from build123d import *

# Parameters (mm, degrees)
BOSS_EXTRUDE1_DEPTH      = 38.735
BOSS_EXTRUDE1_DEPTH_BACK = 38.735
CUT_EXTRUDE4_DEPTH       = 40.625695711


with BuildPart() as part:
    # Sketch1 → Boss-Extrude1 (new, two sides: drawn at the far end of the back side and taken through both)
    with BuildSketch(Plane(origin=(0, 0, 0), x_dir=(1, 0, 0), z_dir=(0, 1, 0)).offset(-BOSS_EXTRUDE1_DEPTH_BACK)):
        with BuildLine():
            Line((2.3876, 4.120773288), (-2.3876, 4.120773288))
            ThreePointArc((-2.3876, 4.120773288), (-2.378072881, -4.126278665), (4.7625, 0))
            ThreePointArc((4.7625, 0), (4.126278665, 2.378072881), (2.3876, 4.120773288))
        make_face()
    extrude(amount=BOSS_EXTRUDE1_DEPTH + BOSS_EXTRUDE1_DEPTH_BACK)

    # Sketch4 → Cut-Extrude4 (cut, through all)
    with BuildSketch(Plane.XY.offset(2.7432)):
        with BuildLine():
            Line((-1.2446, -26.035), (-1.2446, -38.735))
            Line((-1.2446, -38.735), (1.2446, -38.735))
            Line((1.2446, -38.735), (1.2446, -26.035))
            ThreePointArc((1.2446, -26.035), (0, -27.2796), (-1.2446, -26.035))
        make_face()
        with BuildLine():
            ThreePointArc((1.2446, -26.035), (0, -24.7904), (-1.2446, -26.035))
            Line((-1.2446, -26.035), (1.2446, -26.035))
        make_face()
        with BuildLine():
            Line((1.2446, -26.035), (-1.2446, -26.035))
            ThreePointArc((-1.2446, -26.035), (0, -27.2796), (1.2446, -26.035))
        make_face()
        with BuildLine():
            Line((1.2446, 38.735), (-1.2446, 38.735))
            Line((-1.2446, 38.735), (-1.2446, 26.035))
            ThreePointArc((-1.2446, 26.035), (0, 27.2796), (1.2446, 26.035))
            Line((1.2446, 26.035), (1.2446, 38.735))
        make_face()
        with BuildLine():
            ThreePointArc((1.2446, 26.035), (0, 27.2796), (-1.2446, 26.035))
            Line((-1.2446, 26.035), (1.2446, 26.035))
        make_face()
        with BuildLine():
            Line((1.2446, 26.035), (-1.2446, 26.035))
            ThreePointArc((-1.2446, 26.035), (0, 24.7904), (1.2446, 26.035))
        make_face()
    extrude(amount=CUT_EXTRUDE4_DEPTH, mode=Mode.SUBTRACT)


solid = part.part
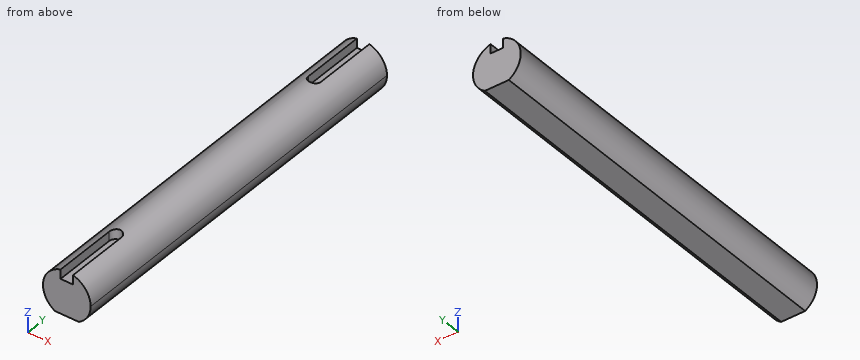
Here's how the part is built. I have some questions about the finished solid (model axes, mm). Round coordinates to 2 decimals unless told otherwise and drop trailing zeros. Loops run counter-clockwise (first coordinate to the right, second up) from the corner with the lowest first, then second, coordinate; pieces in that order, holes last. Notation, with made-up numbers: M -37.75,68.25 L 9.25,68.25 A24 cw 9.25,102.25 Z; hole C -26.75,56 d2. An arc over 180 degrees is marked long. Write each question's results on one line, items separated by ' | '. Start each with the question number.
(1) I want a section at D-D (y = -22.5). Please give me the cut outline in (x, z) (1 decimal).
(2) Will these pins go through, and if not, where does the flat tip stop? P1, Ø2, axis at y = 29.5, z = 1.5, coming from the +X side; P2, Ø1, axis at y = 9.5, z = -1.5, coming from the -X side; P3, Ø0.7, axis at x = 0, y = -33.5, coming from the +Z side.
(3) I want a section at A-A (x = 0). Please give me the cut outline in (y, z) (1 decimal).
(4) If I drill on probe 1 along Z at (x, y) = (-0.5, -34); probe 2 along X at (y, z) = (27, 3.5); probe 3 along Z at (x, y) = (-3, -26.5), over which ranges is the centre line in solid material (lowest first)? Write a range as from..to.
(5) I want a section at B-B (y = 33.5). Please give me the cut outline in (x, z) (1 decimal), then the cut area to 3 significant figures.
(6) I want a section at C-C (z = -2.75). Please give me the cut outline in (x, y) (3 decimals), then the cut area to 3 significant figures.
Solved:
1) outline: M -2.4,-4.1 L 2.4,-4.1 A4.8 ccw long Z
2) P1: stops at x = 4.74 | P2: stops at x = -4.66 | P3: stops at z = 2.74
3) outline: M -38.7,-4.1 L 38.7,-4.1 L 38.7,2.7 L 24.8,2.7 L 24.8,4.8 L -24.8,4.8 L -24.8,2.7 L -38.7,2.7 Z
4) probe 1: z = -4.12..2.74 | probe 2: x = -3.23..-1.24, 1.24..3.23 | probe 3: z = -3.7..3.7
5) outline: M -2.4,-4.1 L 2.4,-4.1 A4.8 ccw 1.2,4.6 L 1.2,2.7 L -1.2,2.7 L -1.2,4.6 A4.8 ccw Z | area: 64.3 mm²
6) outline: M -3.888,-38.735 L 3.888,-38.735 L 3.888,38.735 L -3.888,38.735 Z | area: 602 mm²
